Source: three-view drawing plus pictorial views. Frame: mm from the lowest corner of the part. A direction names the side the tool comes from. Give positions to 0.01 mm unless a question says otherwise; leave off trailing zeros. Order: outer loops, then holes, each group sorted by start corner. A loop starts at its lowest first (then second) coordinate and runs counter-clockwise, first axis right, second up. Notation, with made-up numbers: (8.25, -10.5) -> (47.25, -10.5) arc R25 ccw to (47.25, 11.5) -> close; hole circle Ø6 at (-7, 63). An arc over 180 degrees is marked (long way). Write item = value, one per line.
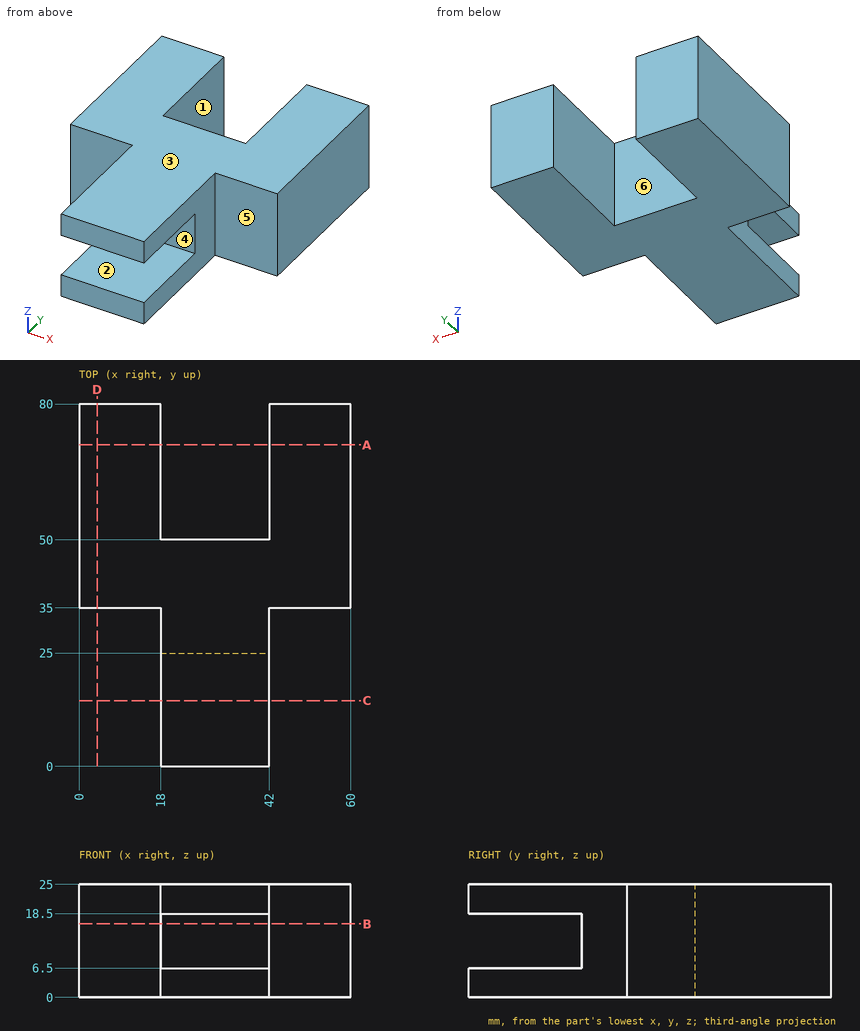
1) First-contact query: P1, Ø5.5, axis at x = 50.5, z = 16, coming from the -Y side; P2, Ø5, axis at y = 12, z = 15.5, coming from the -X side; P3, Ø6, axis at x = 26, z = 14, coming from the -Y side. Flat tips, straight axial feed; report the tip coordinate or a pass-through.
Check sheet entries:
P1 = 35
P2 = through
P3 = 25
2) Section query B-B (z = 16.25). Output: boundary loops of the cut face in (x, y), plus the area to 3 significant figures.
Check sheet entries:
outline = (0, 35) -> (18, 35) -> (18, 25) -> (42, 25) -> (42, 35) -> (60, 35) -> (60, 80) -> (42, 80) -> (42, 50) -> (18, 50) -> (18, 80) -> (0, 80) -> close
area = 2,220 mm²
3) Line query: line 1 (X direction, y = 67, z = 20.75); line 2 (Z direction, x = 28, y = 11.5); line 3 (X direction, y = 28, z = 13). Output: solid intervals per line, ascending. Write a range as from..to.
Check sheet entries:
line_1 = 0..18, 42..60
line_2 = 0..6.5, 18.5..25
line_3 = 18..42
4) Reachability of the marked faces 4, 5 and 6 from +Z, -Z, +X, -X, +Y, -Y: full face, straight path, thin tool, end or side. Return the list, or none.
Check sheet entries:
face_4 = +X, -X, -Y
face_5 = +Z, -Z, +X, -Y
face_6 = +Z, -Z, +Y
5) Section query D-D (x = 4). Output: boundary loops of the cut face in (y, z).
Check sheet entries:
outline = (35, 0) -> (80, 0) -> (80, 25) -> (35, 25) -> close
6) Section query A-A (y = 71). Output: boundary loops of the cut face in (x, z).
Check sheet entries:
outline = (0, 0) -> (18, 0) -> (18, 25) -> (0, 25) -> close; (42, 0) -> (60, 0) -> (60, 25) -> (42, 25) -> close
7) Section query C-C (y = 14.5). Output: boundary loops of the cut face in (x, z), plus the area to 3 significant figures.
Check sheet entries:
outline = (18, 0) -> (42, 0) -> (42, 6.5) -> (18, 6.5) -> close; (18, 18.5) -> (42, 18.5) -> (42, 25) -> (18, 25) -> close
area = 312 mm²
8) Mould query, pull axis Z, two halves, no side actions, for the marked faces 1, 2 and 3. Classes: +Z half, -Z half, draft (parallel to the pull), parting line (faces both ways), or undercut.
Check sheet entries:
face_1 = draft
face_2 = undercut
face_3 = +Z half
